Input: part model. Units: mm. Frame: model coordinates. Coordinates: 2 decimals unless noted, no trailing zeros. Loops run counter-clockwise (first coordinate to the right, second up) from the corner with the lowest first, then second, coordinate; pieces in that order, holes last. Notation, with made-up numbers: (35.25, 54) - (66.25, 54) arc R32 ccw to (66.25, 87) - close; hole circle Ø8 at (1.25, 45). An arc over 180 degrees is marked (long way). Answer as CSV lines item,"result". Start each with the question number.
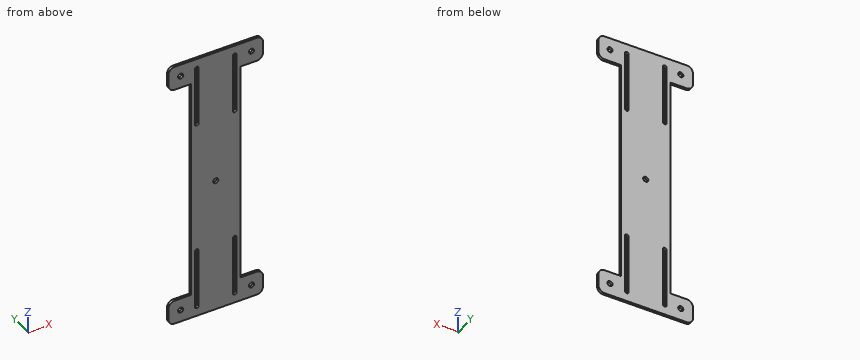
Autodesk Inventor part; units mm, degrees
ref_plane "YZ Plane" through (0, 0, 0) normal (1, 0, 0) x (0, 1, 0)
ref_plane "XZ Plane" through (0, 0, 0) normal (0, 1, 0) x (-1, 0, 0)
ref_plane "XY Plane" through (0, 0, 0) normal (0, 0, 1) x (1, 0, 0)
sketch "Sketch1" plane through (0, 0, 0) normal (0, 1, 0) x (-1, 0, 0)
  line L0 (0, 0) -> (-37.6, 0)
  line L1 (-37.6, -20) -> (-37.6, -51.2)
  line L2 (-37.6, -51.2) -> (0, -51.2)
  line L3 (0, -51.2) -> (0, -20)
  line L4 (-18.8, 0) -> (-1.65, 0)
  line L5 (-1.65, 0) -> (-23.35, 0)
  line L6 (-18.8, 0) -> (5.35, 0)
  line L7 (5.35, 0) -> (-25.85, 0)
  line L8 (-18.8, 0) -> (-3.2, 0)
  line L9 (-3.2, 0) -> (-34.4, 0)
  arc A0 (-32.8, -8.4) -> (-36, -8.4) centre (-34.4, -8.4) ccw
  arc A1 (-36, -46.5) -> (-32.8, -46.5) centre (-34.4, -46.5) ccw
  arc A2 (-1.6, -8.4) -> (-4.8, -8.4) centre (-3.2, -8.4) ccw
  arc A3 (-4.8, -46.5) -> (-1.6, -46.5) centre (-3.2, -46.5) ccw
  line L10 (0, 0) -> (0, -20)
  line L11 (0, -20) -> (20, -20)
  line L12 (20, -20) -> (20, 0)
  line L13 (20, 0) -> (0, 0)
  line L14 (-37.6, -20) -> (-57.6, -20)
  line L15 (-57.6, -20) -> (-57.6, 0)
  line L16 (-57.6, 0) -> (-37.6, 0)
  line L17 (-1.6, -46.5) -> (-1.6, -8.4)
  line L18 (-4.8, -8.4) -> (-4.8, -46.5)
  line L19 (-32.8, -46.5) -> (-32.8, -8.4)
  line L20 (-36, -8.4) -> (-36, -46.5)
  point P0 (5.35, 0)
  dimension "d0" = 37.6
  dimension "d1" = 51.2
  dimension "d41" = 15.6
  dimension "d42" = 31.2
  dimension "d50" = 3.2
  dimension "d56" = 3.2
  dimension "d57" = 3.2
  dimension "d63" = 3.2
  dimension "d67" = 8.4
  dimension "d77" = 8.4
  dimension "d81" = 20
  dimension "d82" = 20
  dimension "d83" = 20
extrude "Extrusion3" add sketch "Sketch1" along normal blind 2
sketch "Sketch2" plane through (0, 2, 0) normal (0, 1, 0) x (1, 0, 0)
  circle A0 centre (-10, 10) radius 2.125
  line L0 (-20, 0) -> (57.6, 0)
  line L1 (38.17, 0) -> (48.17, 0)
  circle A1 centre (48.17, 10) radius 2.125
  point P0 (0, 0)
  dimension "d85" = 4.25
  dimension "d86" = 10
  dimension "d88" = 4.25
extrude "Extrusion4" cut sketch "Sketch2" against normal blind 2
fillet "Fillet3" radius 5 4 edges at (57.6, 1, -20) (57.6, 1, 0) (-20, 1, 0) (-20, 1, -20)
ref_plane "Work Plane2" through (37.6, 0, -112) normal (0, 0, -1) x (-1, 0, 0)
mirror "Mirror2" about plane through (37.6, 0, -112) normal (0, 0, -1)
sketch "Sketch5" plane through (0, 0, 0) normal (0, 1, 0) x (-1, 0, 0)
  line L0 (-37.6, -172.8) -> (0, -172.8)
  line L1 (0, -51.2) -> (-37.6, -51.2)
  line L2 (20, -112) -> (20, -102)
  line L3 (20, -102) -> (0, -102)
  line L4 (20, -112) -> (20, -122)
  line L5 (20, -122) -> (0, -122)
  line L6 (-37.6, -122) -> (-57.6, -122)
  line L7 (-57.6, -122) -> (-57.6, -102)
  line L8 (-57.6, -102) -> (-37.6, -102)
  line L9 (-37.6, -51.2) -> (-37.6, -102)
  line L10 (-37.6, -122) -> (-37.6, -172.8)
  line L11 (0, -172.8) -> (0, -122)
  line L12 (0, -102) -> (0, -51.2)
  circle A0 centre (10, -112) radius 2.125
  circle A1 centre (-47.6, -112) radius 2.125
  point P0 (0, 0)
  dimension "d95" = 10
  dimension "d96" = 10
  dimension "d97" = 20
  dimension "d98" = 4.25
  dimension "d99" = 4.25
extrude "Extrusion5" add sketch "Sketch5" along normal blind 2
fillet "Fillet4" radius 5 4 edges at (57.6, 1, -122) (57.6, 1, -102) (-20, 1, -122) (-20, 1, -102)
sketch "Sketch6" plane through (0, 2, 0) normal (0, 1, 0) x (1, 0, 0)
  arc A0 (4.8, 46.5) -> (1.6, 46.5) centre (3.2, 46.5) ccw
  line L0 (3.2, 46.5) -> (13.2, 46.5) construction
  arc A1 (36, 56.5) -> (32.8, 56.5) centre (34.4, 56.5) ccw
  arc A2 (3.2, 54.9) -> (1.6, 56.5) centre (3.2, 56.5) ccw
  arc A3 (36, 46.5) -> (32.8, 46.5) centre (34.4, 46.5) ccw
  line L1 (36, 46.5) -> (36, 56.5)
  line L2 (32.8, 46.5) -> (32.8, 56.5)
  line L3 (4.8, 46.5) -> (4.8, 56.5)
  line L4 (1.6, 46.5) -> (1.6, 56.5)
  circle A4 centre (34.4, 46.5) radius 1.6
  circle A5 centre (3.2, 46.5) radius 1.6
  point P0 (0, 0)
extrude "Extrusion6" cut sketch "Sketch6" against normal blind 2 contours A0 L4 A2 L3 | L1 A3 L2 A1
sketch "Sketch7" plane through (0, 2, 0) normal (0, 1, 0) x (1, 0, 0)
  arc A0 (1.6, 177.5) -> (4.8, 177.5) centre (3.2, 177.5) ccw
  arc A1 (1.6, 167.5) -> (4.8, 167.5) centre (3.2, 167.5) ccw
  arc A2 (32.8, 167.5) -> (36, 167.5) centre (34.4, 167.5) ccw
  arc A3 (32.8, 177.5) -> (36, 177.5) centre (34.4, 177.5) ccw
  line L0 (36, 177.5) -> (36, 167.5)
  line L1 (32.8, 177.5) -> (32.8, 167.5)
  line L2 (1.6, 177.5) -> (1.6, 167.5)
  line L3 (4.8, 167.5) -> (4.8, 177.5)
  arc A4 (1.6, 177.5) -> (4.8, 177.5) centre (3.2, 177.5) ccw
  arc A5 (32.8, 177.5) -> (36, 177.5) centre (34.4, 177.5) ccw
  point P0 (0, 0)
extrude "Extrusion7" cut sketch "Sketch7" against normal blind 2
sketch "Sketch8" plane through (0, 2, 0) normal (0, 1, 0) x (1, 0, 0)
  line L0 (0, 122) -> (-15, 122)
  line L1 (0, 122) -> (-20, 122)
  line L2 (-20, 122) -> (-20, 102)
  line L3 (-20, 102) -> (0, 102)
  line L4 (0, 102) -> (0, 122)
  point P0 (0, 0)
extrude "Extrusion8" cut sketch "Sketch8" against normal blind 2
sketch "Sketch9" plane through (0, 2, 0) normal (0, 1, 0) x (1, 0, 0)
  line L0 (52.6, 122) -> (37.6, 122)
  line L1 (37.6, 122) -> (57.6, 122)
  line L2 (57.6, 122) -> (57.6, 102)
  line L3 (57.6, 102) -> (37.6, 102)
  line L4 (37.6, 102) -> (37.6, 122)
  point P0 (0, 0)
extrude "Extrusion9" cut sketch "Sketch9" against normal blind 2
sketch "Sketch10" plane through (0, 2, 0) normal (0, 1, 0) x (1, 0, 0)
  line L0 (0, 0) -> (18.8, 0)
  line L1 (-15, 0) -> (52.6, 0)
  line L2 (18.8, 0) -> (18.8, 112)
  circle A0 centre (18.8, 112) radius 2.125
  dimension "d114" = 112
  dimension "d115" = 4.25
extrude "Extrusion10" cut sketch "Sketch10" against normal blind 2
sketch "Sketch11" plane through (0, 2, 0) normal (0, 1, 0) x (1, 0, 0)
  line L0 (0, 20) -> (0, 204)
  line L1 (0, 204) -> (-15, 204)
  line L2 (0, 20) -> (-1.6, 20)
  line L3 (-1.6, 20) -> (-1.6, 204)
  line L4 (-1.6, 204) -> (0, 204)
  line L5 (0, 204) -> (0, 20)
  line L6 (37.6, 20) -> (37.6, 204)
  line L7 (37.6, 204) -> (39.2, 204)
  line L8 (39.2, 204) -> (39.2, 20)
  line L9 (39.2, 20) -> (37.6, 20)
  line L10 (37.6, 20) -> (37.6, 204)
  point P0 (0, 0)
  dimension "d118" = 1.6
  dimension "d119" = 1.6
extrude "Extrusion11" add sketch "Sketch11" against normal blind 2
properties part number "Motor Attachment 2.0"
Item 1: Material intervals for probe 1 along X at (y, z) = (0.35, -44.5); probe 2 along Z at (x, y) = (-10, 0.95) (3 decimals); probe 3 along Z at (x, y) = (33, 1.4), sorted ascending.
Item 2: Section query D-D, the plane z = -133.5. Output: boundary loops of the cut face in (x, y).
Item 3: Section query C-C, the plane y = 1.5. Give the number of separate pieces and of enclosed holes in the cut face, and give its area (3 significant figures).
Item 4: Section query B-B, the plane x = 48.17. Output: boundary loops of the cut face in (y, z) (3 decimals).
Item 5: Section query A-A, the plane z = -32. Output: boundary loops of the cut face in (x, y).
Item 6: Contact query for flat-ended pins moving along their axis: P1, Ø0.6, axis at y = 1, z = -184, coming from the +X side; P2, Ø0.6, axis at y = 1, z = -22, coming from the -X side; P3, Ø3.5, axis at x = -10, z = -10, coming from the -Y side. Output: stop coordinate, or through.
Response values:
1,probe 1,"x = -1.6 to 1.6, 4.8 to 32.8, 36 to 39.2"
1,probe 2,"z = -224 to -216.125, -211.875 to -204, -20 to -12.125, -7.875 to 0"
1,probe 3,"z = -224 to -216.37, -166.73 to -57.27, -7.63 to 0"
2,outline,"(-1.6, 0) - (39.2, 0) - (39.2, 2) - (-1.6, 2) - close"
3,separate pieces,"1"
3,enclosed holes,"9"
3,area,"9,850 mm²"
4,outline,"(0, -224) - (2, -224) - (2, -216.125) - (0, -216.125) - close; (0, -211.875) - (2, -211.875) - (2, -204) - (0, -204) - close; (0, -20) - (2, -20) - (2, -12.125) - (0, -12.125) - close; (0, -7.875) - (2, -7.875) - (2, 0) - (0, 0) - close"
5,outline,"(-1.6, 0) - (1.6, 0) - (1.6, 2) - (-1.6, 2) - close; (4.8, 0) - (32.8, 0) - (32.8, 2) - (4.8, 2) - close; (36, 0) - (39.2, 0) - (39.2, 2) - (36, 2) - close"
6,P1,"stops at x = 39.2"
6,P2,"stops at x = -1.6"
6,P3,"passes through"
